Part model, mm, in its own coordinate system. Round coordinates to 2 decimals unless told otherwise and drop trailing zeros. Order: outer loops, then holes, each group sorted by start corner. A loop starts at its lowest first (then second) coordinate and runs counter-clockwise, first axis right, second up. Notation, with made-up numbers: M -38.75,79.25 L -17.75,79.25 A21 ccw -17.75,97.25 Z; hole C 9.5,83.25 d2. An arc over 180 degrees is marked long. Write each question's results on one line, items separated by ' | '. Start each with the question number.
1. Probe L1, parallel to Z at x = -21, y = -1.45; L2, parallel to Y at x = -14, z = -5.5. List the from-to ranges inside material, lowest first. Write a range as [from, to].
2. Drop a flat-ended pin along its axis: pin 1 Ø1 at (x, z) = (-27.5, 6.5) entering from +Y. Give the stop position or say it passes through.
3. Band-saw the part on B-B, the plane y = -1.3. Give the number of separate pieces and of enclosed holes in the cut face, then the cut area to 3 significant figures.
4. Band-saw the part on A-A, the plane x = -27. List the corners of the cut face in (y, z).
Autodesk Inventor part; units mm, degrees
ref_plane "YZ Plane" through (0, 0, 0) normal (1, 0, 0) x (0, 1, 0)
ref_plane "XZ Plane" through (0, 0, 0) normal (0, 1, 0) x (-1, 0, 0)
ref_plane "XY Plane" through (0, 0, 0) normal (0, 0, 1) x (1, 0, 0)
sketch "Sketch1" plane through (0, 0, 0) normal (0, 1, 0) x (-1, 0, 0)
  line L0 (28.6, -28) -> (25.4, -28)
  line L1 (25.4, -28) -> (25.4, 28)
  line L2 (25.4, 28) -> (28.6, 28)
  line L3 (28.6, 28) -> (28.6, -28)
  line L4 (28.6, -28) -> (25.4, 28) construction
  line L5 (25.4, -28) -> (28.6, 28) construction
  line L6 (22.6, -28) -> (19.4, -28)
  line L7 (19.4, -28) -> (19.4, 28)
  line L8 (19.4, 28) -> (22.6, 28)
  line L9 (22.6, 28) -> (22.6, -28)
  line L10 (22.6, -28) -> (19.4, 28) construction
  line L11 (19.4, -28) -> (22.6, 28) construction
  line L12 (16.6, -28) -> (13.4, -28)
  line L13 (13.4, -28) -> (13.4, 28)
  line L14 (13.4, 28) -> (16.6, 28)
  line L15 (16.6, 28) -> (16.6, -28)
  line L16 (16.6, -28) -> (13.4, 28) construction
  line L17 (13.4, -28) -> (16.6, 28) construction
  line L18 (10.6, -28) -> (7.4, -28)
  line L19 (7.4, 28) -> (10.6, 28)
  line L20 (7.4, -28) -> (7.4, 28)
  line L21 (10.6, -28) -> (7.4, 28) construction
  line L22 (7.4, -28) -> (10.6, 28) construction
  line L23 (10.6, 28) -> (10.6, -28)
  line L24 (4.6, -28) -> (1.4, -28)
  line L25 (1.4, 28) -> (4.6, 28)
  line L26 (1.4, -28) -> (1.4, 28)
  line L27 (4.6, -28) -> (1.4, 28) construction
  line L28 (1.4, -28) -> (4.6, 28) construction
  line L29 (4.6, 28) -> (4.6, -28)
  line L30 (-1.4, -28) -> (-4.6, -28)
  line L31 (-4.6, 28) -> (-1.4, 28)
  line L32 (-4.6, -28) -> (-4.6, 28)
  line L33 (-1.4, -28) -> (-4.6, 28) construction
  line L34 (-4.6, -28) -> (-1.4, 28) construction
  line L35 (-1.4, 28) -> (-1.4, -28)
  line L36 (-7.4, 28) -> (-7.4, -28)
  line L37 (-10.6, -28) -> (-7.4, 28) construction
  line L38 (-10.6, -28) -> (-10.6, 28)
  line L39 (-7.4, -28) -> (-10.6, 28) construction
  line L40 (-10.6, 28) -> (-7.4, 28)
  line L41 (-7.4, -28) -> (-10.6, -28)
  line L42 (-13.4, 28) -> (-13.4, -28)
  line L43 (-16.6, -28) -> (-13.4, 28) construction
  line L44 (-16.6, -28) -> (-16.6, 28)
  line L45 (-13.4, -28) -> (-16.6, 28) construction
  line L46 (-16.6, 28) -> (-13.4, 28)
  line L47 (-13.4, -28) -> (-16.6, -28)
  line L48 (-19.4, 28) -> (-19.4, -28)
  line L49 (-22.6, -28) -> (-19.4, 28) construction
  line L50 (-22.6, -28) -> (-22.6, 28)
  line L51 (-19.4, -28) -> (-22.6, 28) construction
  line L52 (-22.6, 28) -> (-19.4, 28)
  line L53 (-19.4, -28) -> (-22.6, -28)
  line L54 (-25.4, 28) -> (-25.4, -28)
  line L55 (-28.6, -28) -> (-25.4, 28) construction
  line L56 (-28.6, -28) -> (-28.6, 28)
  line L57 (-25.4, -28) -> (-28.6, 28) construction
  line L58 (-28.6, 28) -> (-25.4, 28)
  line L59 (-25.4, -28) -> (-28.6, -28)
  line L60 (0, 0) -> (33.435, 0)
  point P0 (27, 28)
  point P1 (21, 28)
  point P2 (15, 28)
  point P3 (9, 28)
  point P4 (3, 28)
  point P5 (-3, 28)
  point P6 (-9, 28)
  point P7 (-15, 28)
  point P8 (-21, 28)
  point P9 (-27, 28)
  point P10 (27, -28)
  point P11 (21, 0)
  point P12 (27, 0)
  point P13 (15, 0)
  point P14 (21, 0)
  point P15 (9, 0)
  point P16 (15, 0)
  point P17 (3, 0)
  point P18 (9, 0)
  point P19 (-3, 0)
  point P20 (3, 0)
  point P21 (-9, 0)
  point P22 (-3, 0)
  point P23 (-15, 0)
  point P24 (-9, 0)
  point P25 (-21, 0)
  point P26 (-15, 0)
  point P27 (-27, 0)
  point P28 (-21, 0)
  point P29 (27, 0)
  dimension "d0" = 3.2
  dimension "d1" = 3.2
  dimension "d2" = 3.2
  dimension "d3" = 3.2
  dimension "d4" = 3.2
  dimension "d5" = 3.2
  dimension "d6" = 3.2
  dimension "d7" = 3.2
  dimension "d8" = 3.2
  dimension "d9" = 6
  dimension "d10" = 6
  dimension "d11" = 6
  dimension "d12" = 6
  dimension "d13" = 6
  dimension "d14" = 6
  dimension "d15" = 6
  dimension "d16" = 6
  dimension "d17" = 6
  dimension "d19" = 3
  dimension "d26" = 56
sketch "Sketch2" plane through (0, 0, 0) normal (0, 1, 0) x (-1, 0, 0)
  line L0 (-30.6, -30.2) -> (30.6, -30.2)
  line L1 (30.6, -30.2) -> (30.6, 30.2)
  line L2 (30.6, 30.2) -> (-30.6, 30.2)
  line L3 (-30.6, 30.2) -> (-30.6, -30.2)
  line L4 (-30.6, -30.2) -> (30.6, 30.2) construction
  line L5 (30.6, -30.2) -> (-30.6, 30.2) construction
  point P0 (0, 0)
  dimension "d20" = 60.4
  dimension "d21" = 61.2
extrude "Extrusion1" add sketch "Sketch2" against normal blind 5
extrude "Extrusion2" cut sketch "Sketch1" against normal blind 3.5
equation "\"d1\" = d0"
equation "\"d2\" = d0"
equation "\"d3\" = d0"
equation "\"d4\" = d0"
equation "\"d5\" = d4"
equation "\"d6\" = d5"
equation "\"d7\" = d6"
equation "\"d8\" = d6"
properties part number "DisplayModuleHousingCap"
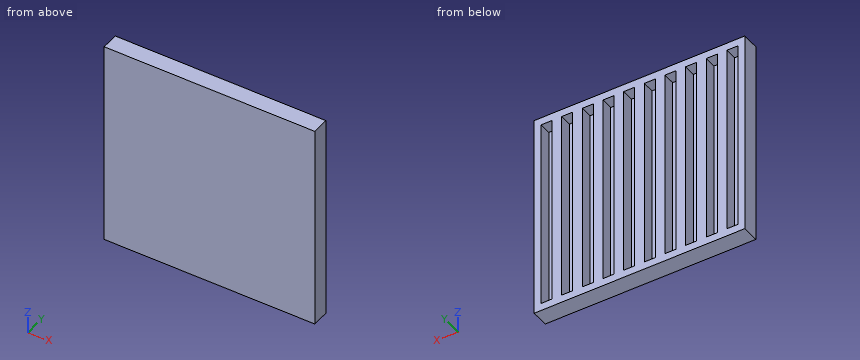
Solution:
1) L1: [-30.2, -28], [28, 30.2] | L2: [-5, -3.5]
2) pin 1: y = -3.5
3) separate pieces: 1 | enclosed holes: 10 | area: 1,900 mm^2
4) outline: M -5,-30.2 L 0,-30.2 L 0,-28 L -3.5,-28 L -3.5,28 L 0,28 L 0,30.2 L -5,30.2 Z
